The figure shows three views and two pictorial views of one solid part (mm, origin at its lowest corner). Answer the questions. A direction names the side the tool comes from. Coordinates: 2 decimals unless noted, no trailing zeros. Order: outer loops, then holes, each group sorted by start corner. A loop starts at its lowest first (then second) coordinate and runs counter-clockwise, first axis right, second up. Notation, with made-up numbers: (87, -33.5) -> (95, -33.5) arc R23 cw to (95, -13.5) -> close; hole circle Ø5 at (-32.75, 76). An arc over 180 degrees is marked (long way). Write item = value, one per line. Start each with the question number.
Q1. The part is cut by section A-A, the plane y = 1.65. Count the separate pieces of the cut face and the enclosed holes in it, plus the area to 3 significant figures.
Q2. Which of the six approach directions +Z, -Z, +X, -X, +Y, -Y give full straight-line access (tool end or side, diameter ignored) to the marked faces 4 and 5?
Q3. For a pull along Z with two mould halves and no side action, classify the marked faces 1, 2 and 3 as +Z half, -Z half, draft (parallel to the pull), parting line (faces both ways), or undercut.
Q4. Flat-ended cylindrical pins translate along their axes: pin 1 (7 mm diameter, centred on x = 7, z = 5.5, fed in from +Y); pin 2 (2 mm diameter, centred on x = 6, y = 4.5, fed in from +Z); pin 3 (1.8 mm diameter, centred on x = 16.51, z = 10.16, fed in from -Y). Find the tip coordinate at first contact, or state that the pin passes through.
Q5. The part is cut by section B-B, the plane x = 6.35. Determine the outline of the cut face in (y, z).
Q6. The part is cut by section C-C, the plane y = 4.5. Determine the outline of the cut face in (x, z) (1 decimal).
Q7. Straight lines are drawn through the part: L1, parallel to X at y = 3.5, z = 11 (1 decimal); L2, parallel to X at y = 0.6, z = 10.16; L3, parallel to Z at x = 16.51, y = 1.7. For each, find the intervals that lie inside material, in ascending order. Write a range as from..to.
Q8. The part is cut by section D-D, the plane z = 10.16. Determine the outline of the cut face in (x, y) (1 decimal).
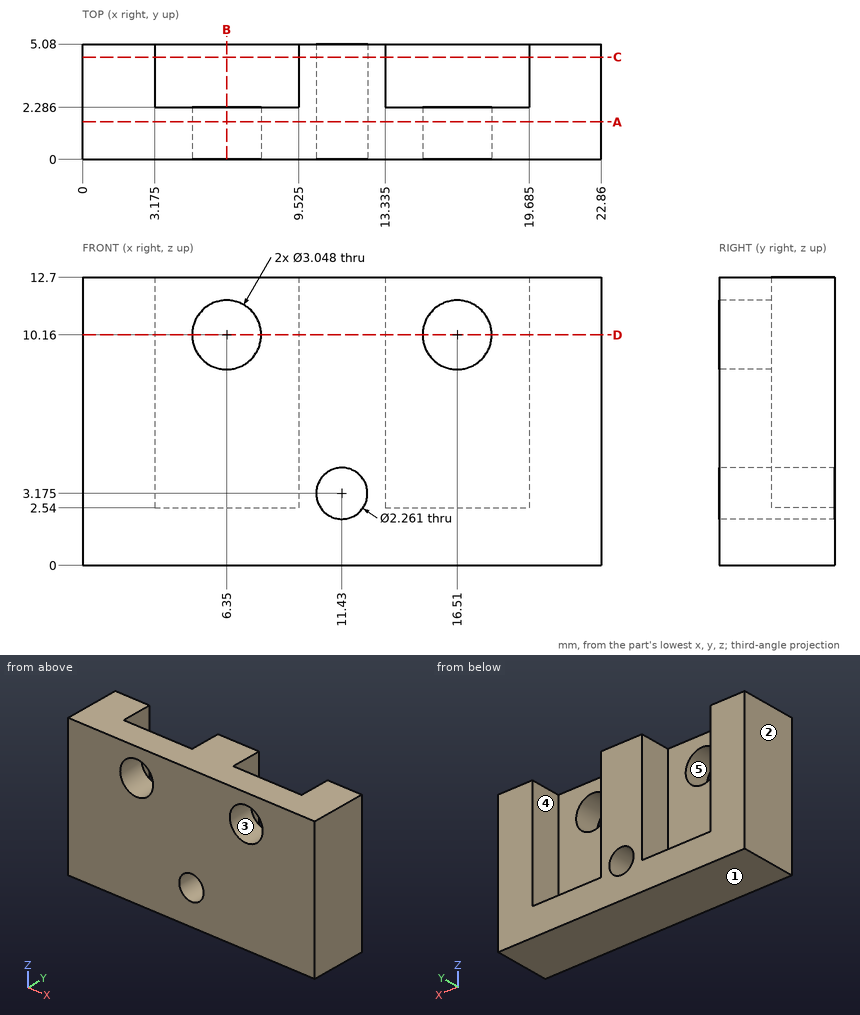
Model answer:
q1.separate_pieces = 1
q1.enclosed_holes = 3
q1.area = 272 mm2
q2.face_4 = +Z, +Y
q2.face_5 = +Y, -Y
q3.face_1 = -Z half
q3.face_2 = draft
q3.face_3 = undercut
q4.pin_1 = 5.08
q4.pin_2 = 2.54
q4.pin_3 = through
q5.outline = (0, 0) -> (5.08, 0) -> (5.08, 2.54) -> (2.29, 2.54) -> (2.29, 8.64) -> (0, 8.64) -> close; (0, 11.68) -> (2.29, 11.68) -> (2.29, 12.7) -> (0, 12.7) -> close
q6.outline = (0, 0) -> (22.9, 0) -> (22.9, 12.7) -> (19.7, 12.7) -> (19.7, 2.5) -> (13.3, 2.5) -> (13.3, 12.7) -> (9.5, 12.7) -> (9.5, 2.5) -> (3.2, 2.5) -> (3.2, 12.7) -> (0, 12.7) -> close; hole circle Ø2.3 at (11.4, 3.2)
q7.L1 = 0..3.2, 9.5..13.3, 19.7..22.9
q7.L2 = 0..4.83, 7.87..14.99, 18.03..22.86
q7.L3 = 0..8.64, 11.68..12.7
q8.outline = (0, 0) -> (4.8, 0) -> (4.8, 2.3) -> (3.2, 2.3) -> (3.2, 5.1) -> (0, 5.1) -> close; (7.9, 0) -> (15, 0) -> (15, 2.3) -> (13.3, 2.3) -> (13.3, 5.1) -> (9.5, 5.1) -> (9.5, 2.3) -> (7.9, 2.3) -> close; (18, 0) -> (22.9, 0) -> (22.9, 5.1) -> (19.7, 5.1) -> (19.7, 2.3) -> (18, 2.3) -> close
